For this review, take the finished solid that the model builds, in its own axes (mm). Face numbers are marked on the shaded views. Coordinates: 2 decimals unless noted, no trailing zeros. Write each loop counter-clockwise with the first axis right and the second up, starting at its lowest first coordinate (ties: lowest second). Pieces come first, ordered by that corner, then holes.
1) We need section C-C on y = -14. Write out the cut boundary in (x, z), then the cut area to 3 significant figures.
2) Insertion check: P1, Ø17.5, axis at x = 119.06, y = -68.74, coming from the +Z side. The pin has a flat end and moves straight along its axis. Give the tip position at first contact, or say it passes through.
3) We need section B-B on z = 1.1. Write out the cut boundary in (x, y).
4) Mouldability with a two-part tool opening along Z and no side actions: class the marked faces 1 and 2 as pulls with the +Z half, pulls with the -Z half, needs draft (parallel to the pull), parting line crosses it, or undercut.
5) To check wall thickness, follow line 1 along Y through (x, z) = (121, 0.7); line 2 along X through (y, z) = (139, 2.7); line 3 along X through (y, z) = (-42.5, 3.7). State the ranges of each line that lie inside material, in increasing order.
6) We need section A-A on x = 0. Write out the cut boundary in (y, z).
7) We need section D-D on x = 145. Write out the cut boundary in (y, z), then the cut area to 3 significant figures.
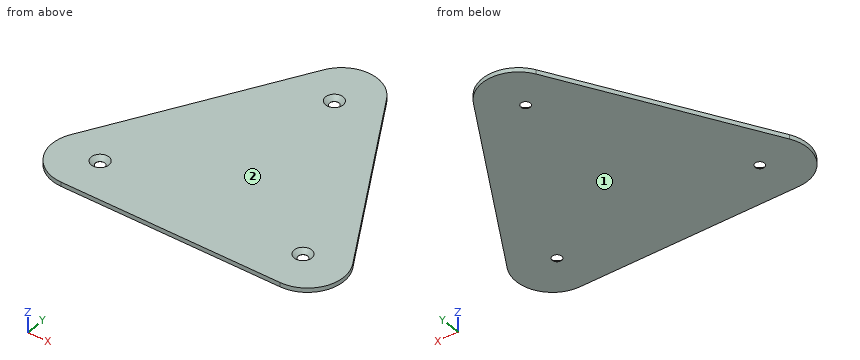
from build123d import *

# Parameters (mm, degrees)
BOSS_EXTRUDE1_DEPTH                           = 5.08
CSK_FOR_M10_FLAT_HEAD_MACHINE_SCREW1_AT_COUNT = 2
CSK_FOR_M10_FLAT_HEAD_MACHINE_SCREW1_AT_PITCH = 238.125
CSK_FOR_M10_FLAT_HEAD_MACHINE_SCREW1_2_COUNT  = 2
CSK_FOR_M10_FLAT_HEAD_MACHINE_SCREW1_2_PITCH  = 238.125


with BuildPart() as part:
    # Sketch1 → Boss-Extrude1 (new body)
    with BuildSketch(Plane.XY):
        with BuildLine():
            Line((-128.5875, -116.86748613), (128.5875, -116.86748613))
            ThreePointArc((128.5875, -116.86748613), (165.503961865, -95.553756935), (165.503961865, -52.926298544))
            Line((165.503961865, -52.926298544), (36.916461865, 169.793784674))
            ThreePointArc((36.916461865, 169.793784674), (0, 191.10751387), (-36.916461865, 169.793784674))
            Line((-36.916461865, 169.793784674), (-165.503961865, -52.926298544))
            ThreePointArc((-165.503961865, -52.926298544), (-165.503961865, -95.553756935), (-128.5875, -116.86748613))
        make_face()
    extrude(amount=BOSS_EXTRUDE1_DEPTH)

    # Sketch3 → CSK for M10 Flat Head Machine Screw1 (revolve, cut)
    with BuildSketch(Plane(origin=(0, 137.481532851, 5.08), x_dir=(0, -1, 0), z_dir=(1, 0, 0))):
        Polygon((0, 0), (0, 5.08), (5.5, 5.08), (5.5, 4.881), (10.381, 0), align=None)
    csk_for_m10_flat_head_machine_screw1 = revolve(axis=Axis((0, 137.481532851, 11.43), (0, 0, -1)), mode=Mode.SUBTRACT)

    # CSK for M10 Flat Head Machine Screw1 at: CSK for M10 Flat Head Machine Screw1 ×2
    with Locations(*[Vector(-0.5, -0.8660254037844387, 0) * (i * CSK_FOR_M10_FLAT_HEAD_MACHINE_SCREW1_AT_PITCH) for i in range(1, CSK_FOR_M10_FLAT_HEAD_MACHINE_SCREW1_AT_COUNT)]):
        add(csk_for_m10_flat_head_machine_screw1, mode=Mode.SUBTRACT)

    # CSK for M10 Flat Head Machine Screw1 2: CSK for M10 Flat Head Machine Screw1 ×2
    with Locations(*[Vector(0.5, -0.8660254037844387, 0) * (i * CSK_FOR_M10_FLAT_HEAD_MACHINE_SCREW1_2_PITCH) for i in range(1, CSK_FOR_M10_FLAT_HEAD_MACHINE_SCREW1_2_COUNT)]):
        add(csk_for_m10_flat_head_machine_screw1, mode=Mode.SUBTRACT)


solid = part.part
Result:
1. outline: (-143.03, 0) - (143.03, 0) - (143.03, 5.08) - (-143.03, 5.08) - close
1. area: 1,450 mm2
2. P1: stops at z = 3.45
3. outline: (-165.5, -52.93) arc R42.63 ccw to (-128.59, -116.87) - (128.59, -116.87) arc R42.63 ccw to (165.5, -52.93) - (36.92, 169.79) arc R42.63 ccw to (-36.92, 169.79) - close; hole circle Ø12.8 at (-119.06, -68.74); hole circle Ø12.8 at (0, 137.48); hole circle Ø12.8 at (119.06, -68.74)
4. face 1: pulls with the -Z half
4. face 2: pulls with the +Z half
5. line 1: y = -116.87 to -74.42, -63.06 to 24.16
5. line 2: x = -54.7 to -7.86, 7.86 to 54.7
5. line 3: x = -159.48 to 159.48
6. outline: (-116.87, 0) - (131.98, 0) - (131.98, 0.2) - (127.1, 5.08) - (-116.87, 5.08) - close; (142.98, 0) - (191.11, 0) - (191.11, 5.08) - (147.86, 5.08) - (142.98, 0.2) - close
7. outline: (-113.58, 0) - (-17.41, 0) - (-17.41, 5.08) - (-113.58, 5.08) - close
7. area: 489 mm2
